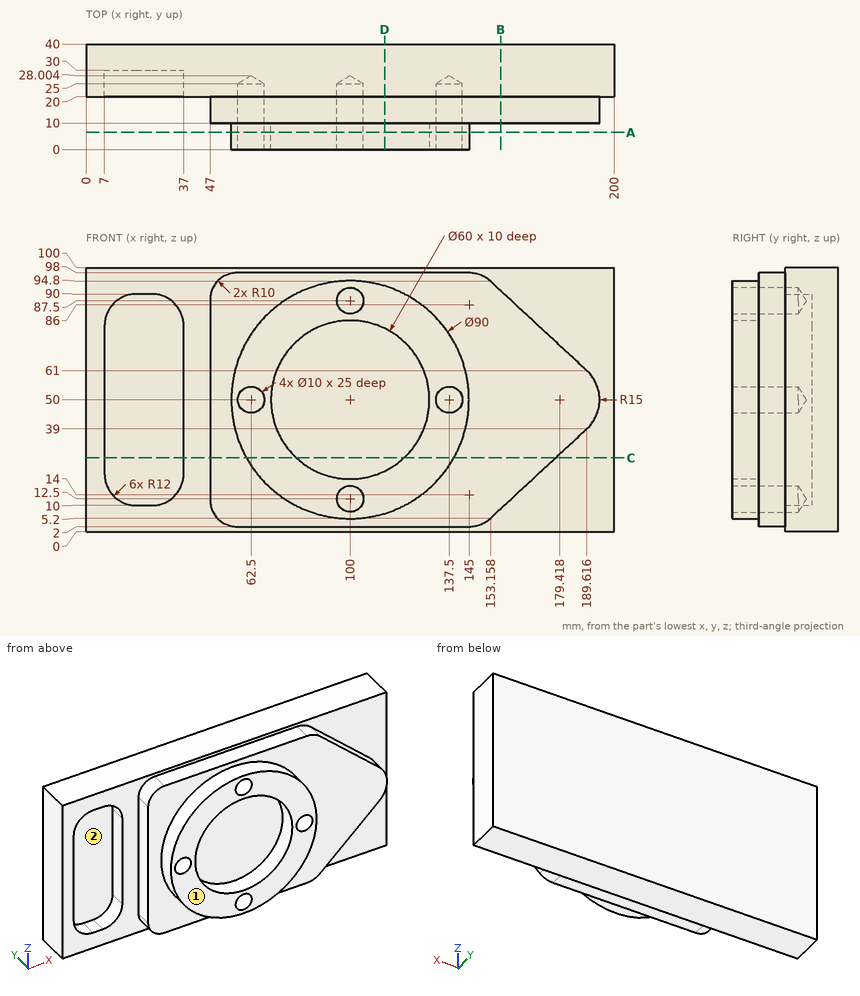
Source: three-view drawing plus pictorial views. Frame: mm from the lowest corner of the part. A direction names the side the tool comes from. Coordinates: 2 decimals unless noted, no trailing zeros. Loops run counter-clockwise (first coordinate to the right, second up) from the corner with the lowest first, then second, coordinate; pieces in that order, holes last. Notation, with made-up numbers: (-39.75, -8) -> (16.25, -8) arc R10 cw to (16.25, 8) -> close; hole circle Ø8 at (-36.75, -18). An arc over 180 degrees is marked (long way). One line per item, written item: value.
(1) Ray query, line 1 along X through (y, z) = (15, 50); line 2 along Z through (x, y) = (62.5, 14); line 3 along Z through (x, y) = (96.5, 8) (1 decimal). Return the intervals inside material, ascending.
Answer below:
line 1: x = 47 to 57.5, 67.5 to 132.5, 142.5 to 194.42
line 2: z = 2 to 45, 55 to 98
line 3: z = 5.1 to 8.9, 16.1 to 20.2, 79.8 to 83.9, 91.1 to 94.9
(2) Cut plane C-C (z = 28). Output: boundary loops of the cut face in (x, y) (1 decimal).
Answer below:
outline: (0, 20) -> (7, 20) -> (7, 30) -> (37, 30) -> (37, 20) -> (47, 20) -> (47, 10) -> (60.7, 10) -> (60.7, 0) -> (79.6, 0) -> (79.6, 10) -> (120.4, 10) -> (120.4, 0) -> (139.3, 0) -> (139.3, 10) -> (177.8, 10) -> (177.8, 20) -> (200, 20) -> (200, 40) -> (0, 40) -> close
(3) Set-up query: the marked faces 1 and 2. Return all of +Z, -Z, +X, -X, +Y, -Y with unobstructed straight access to the full face (end or side cutting, diameter ignored); none if empty.
Answer below:
face 1: +Z, -Z, +X, -X, -Y
face 2: -Y
(4) Cut plane B-B (x = 157). Output: boundary loops of the cut face in (y, z), then the cut area to 4 significant figures.
Answer below:
outline: (10, 8.76) -> (20, 8.76) -> (20, 0) -> (40, 0) -> (40, 100) -> (20, 100) -> (20, 91.24) -> (10, 91.24) -> close
area: 2,825 mm2
(5) Pin query (flat end, axial travel): pin 1 Ø3 at (y, z) = (15, 46.5) entering from -X; pin 2 Ø3 at (x, y) = (22.5, 26) entering from -Z; pin 3 Ø15 at (x, z) = (24, 40.5) entering from -Y; pin 4 Ø5 at (x, y) = (102, 12.5) entering from +Z. Return the tip coordinate at first contact, or that it passes through.
Answer below:
pin 1: stops at x = 47
pin 2: stops at z = 0
pin 3: stops at y = 30
pin 4: stops at z = 98
(6) Cut plane A-A (y = 6.5). Output: boundary loops of the cut face in (x, z), then the cut area to 3 significant figures.
Answer below:
outline: circle Ø90 at (100, 50); hole circle Ø10 at (62.5, 50); hole circle Ø60 at (100, 50); hole circle Ø10 at (100, 12.5); hole circle Ø10 at (100, 87.5); hole circle Ø10 at (137.5, 50)
area: 3,220 mm2
(7) Cut plane D-D (x = 113). Output: boundary loops of the cut face in (y, z).
Answer below:
outline: (0, 6.92) -> (10, 6.92) -> (10, 2) -> (20, 2) -> (20, 0) -> (40, 0) -> (40, 100) -> (20, 100) -> (20, 98) -> (10, 98) -> (10, 93.08) -> (0, 93.08) -> (0, 77.04) -> (10, 77.04) -> (10, 22.96) -> (0, 22.96) -> close
